Autodesk Inventor part; units mm, degrees
ref_plane "Work Plane1" through (0, 0, 26.65) normal (0, 0, 1) x (1, 0, 0)
ref_plane "YZ Plane" through (0, 0, 0) normal (1, 0, 0) x (0, 1, 0)
ref_plane "XZ Plane" through (0, 0, 0) normal (0, 1, 0) x (-1, 0, 0)
sketch "Sketch1" plane through (0, 0, 0) normal (1, 0, 0) x (0, 1, 0)
  line L0 (0, 0) -> (0, -22.65)
  line L1 (0, 0) -> (0, 26.65)
  line L2 (4, -26.65) -> (51, -26.65)
  arc A0 (0, -22.65) -> (4, -26.65) centre (4, -22.65) ccw
  point P0 (0, -26.65)
  dimension "d0" = 26.65
  dimension "d1" = 26.65
  dimension "d2" = 51
  dimension "d3" = 4
ref_plane "Work Plane1" through (0, 0, 26.65) normal (0, 0, 1) x (1, 0, 0)
sketch "Sketch2" plane through (0, 0, 26.65) normal (0, 0, 1) x (1, 0, 0)
  line L0 (-25, 1.5) -> (25, 1.5)
  line L1 (25, 1.5) -> (25, -1.5)
  line L2 (25, -1.5) -> (-25, -1.5)
  line L3 (-25, -1.5) -> (-25, 1.5)
  line L4 (-25, 1.5) -> (25, -1.5) construction
  line L5 (25, 1.5) -> (-25, -1.5) construction
  point P0 (0, 0)
  dimension "d4" = 50
  dimension "d5" = 3
sweep "Sweep1" add profiles "Sketch2" path "Sketch1"
sketch "Sketch3" plane through (25, 4, -28.15) normal (0, 0, -1) x (-1, 0, 0)
  line L0 (0, 47) -> (50, 47) construction
  line L1 (50, 0) -> (50, 47) construction
  circle A0 centre (25, 26.5) radius 11
  point P0 (25, -4)
  dimension "d8" = 22
  dimension "d9" = 20.5
  dimension "d10" = 25
extrude "Extrusion1" cut sketch "Sketch3" against normal blind 10
sketch "Sketch4" plane through (25, 4, -28.15) normal (0, 0, -1) x (-1, 0, 0)
  circle A0 centre (25, 26.5) radius 11 construction
  line L0 (50, 0) -> (50, 47) construction
  line L1 (0, 0) -> (0, 47) construction
  line L2 (0, 47) -> (50, 47) construction
  line L3 (0, 0) -> (50, 0) construction
  circle A1 centre (40.5, 42) radius 2
  line L4 (25, 26.5) -> (14, 26.5) construction
  circle A2 centre (25, 26.5) radius 11 construction
  line L5 (25, 26.5) -> (25, 15.5) construction
  circle A3 centre (9.5, 42) radius 2
  circle A4 centre (40.5, 11) radius 2
  circle A5 centre (9.5, 11) radius 2
  line L6 (25, 26.5) -> (40.5, 42) construction
  circle A6 centre (35.253, 36.753) radius 2
  circle A7 centre (14.747, 36.753) radius 2
  circle A8 centre (35.253, 16.247) radius 2
  circle A9 centre (14.747, 16.247) radius 2
  point P0 (25, -4)
  point P1 (33.8388, 35.3388)
  point P2 (32.7782, 34.2782)
  dimension "d17" = 4
  dimension "d13" = 4
  dimension "d14" = 15.5
  dimension "d15" = 15.5
  dimension "d18" = 1.5
extrude "Extrusion2" cut sketch "Sketch4" against normal blind 10
sketch "Sketch5" plane through (25, 4, -28.15) normal (0, 0, -1) x (-1, 0, 0)
  line L0 (0, 47) -> (50, 47) construction
  line L1 (50, 0) -> (50, 47) construction
  line L2 (0, 0) -> (0, 47) construction
  line L3 (0, 43.5) -> (5, 47)
  line L4 (25, 47) -> (25, 37.5) construction
  circle A0 centre (25, 26.5) radius 11 construction
  line L5 (50, 43.5) -> (45, 47)
  line L6 (0, 43.5) -> (0, 47)
  line L7 (0, 47) -> (5, 47)
  line L8 (45, 47) -> (50, 47)
  line L9 (50, 47) -> (50, 43.5)
  line L10 (50, 0) -> (50, 47)
  point P0 (25, -4)
  point P1 (0, 23.5)
  dimension "d21" = 20
  dimension "d22" = 20
extrude "Extrusion3" cut sketch "Sketch5" against normal blind 10
sketch "Sketch6" plane through (-25, 1.5, 26.65) normal (0, 1, 0) x (1, 0, 0)
  line L0 (0, 0) -> (0, 49.3) construction
  line L1 (0, 0) -> (50, 0) construction
  line L2 (50, 0) -> (50, 49.3) construction
  line L3 (45, 0) -> (50, 4.65)
  line L4 (25, 0) -> (25, 26.65) construction
  line L5 (5, 0) -> (0, 4.65)
  line L6 (5, 0) -> (0, 0)
  line L7 (0, 4.65) -> (0, 0)
  line L8 (45, 0) -> (50, 0)
  line L9 (50, 4.65) -> (50, 0)
  point P0 (50, 24.65)
  dimension "d25" = 20
  dimension "d26" = 20
extrude "Extrusion4" cut sketch "Sketch6" against normal blind 10
sketch "Sketch7" plane through (-25, 1.5, -22.65) normal (0, 1, 0) x (1, 0, 0)
  line L0 (10, -40.3) -> (10, -6.3) construction
  line L1 (12, -38.3) -> (12, -8.3)
  line L2 (8, -8.3) -> (8, -38.3)
  arc A0 (8, -38.3) -> (12, -38.3) centre (10, -38.3) ccw
  arc A1 (12, -8.3) -> (8, -8.3) centre (10, -8.3) ccw
  line L3 (11.5, 2.5) -> (7.5, 2.5) construction
  line L4 (0, -44.65) -> (0, 0) construction
  line L5 (45, -49.3) -> (5, -49.3) construction
  line L6 (25, -49.3) -> (25, -22.65) construction
  line L7 (38, -38.3) -> (38, -8.3)
  line L8 (42, -8.3) -> (42, -38.3)
  arc A2 (38, -38.3) -> (42, -38.3) centre (40, -38.3) ccw
  arc A3 (42, -8.3) -> (38, -8.3) centre (40, -8.3) ccw
  point P0 (10, -23.3)
  dimension "d29" = 34
  dimension "d30" = 4
  dimension "d31" = 8
  dimension "d32" = 9
extrude "Extrusion5" cut sketch "Sketch7" against normal blind 10
fillet "Fillet1" radius 1 8 edges at (20, 51, -26.65) (-20, 51, -26.65) (-25, 47.5, -26.65) (25, 47.5, -26.65) (25, 0, 22) (20, 0, 26.65) (-20, 0, 26.65) (-25, 0, 22)
sketch "Sketch8" plane through (-25, 4, -25.15) normal (-1, 0, 0) x (0, 0, 1)
  line L0 (0, 0) -> (0, 42.9793)
  arc A0 (0, 0) -> (2.5, -2.5) centre (2.5, 0) ccw
  line L1 (46.7144, -2.5) -> (2.5, -2.5)
  line L2 (10.8, -2.5) -> (40.8, -2.5)
  line L3 (0, 19.9793) -> (16.7144, -2.5)
  point P0 (25.15, -4)
  dimension "d36" = 30
  dimension "d37" = 23
extrude "Extrusion6" add sketch "Sketch8" against normal blind 2.5
mirror "Mirror1" about plane through (0, 0, 0) normal (1, 0, 0) of "Extrusion6"
properties part number "Stepper Bracket"
Can you work these out from the model? Positions are in its coordinate system, mm. A direction names the side the tool comes from. Give positions to 0.01 mm unless a question says otherwise; leave off trailing zeros. Order: outer loops, then holes, each group sorted by start corner. A loop starts at its lowest first (then second) coordinate and runs counter-clockwise, first axis right, second up. Notation, with made-up numbers: (-19.5, -10) - (14.5, -10) arc R33 cw to (14.5, 20) - close; hole circle Ø9 at (46.5, 10.5). An arc over 180 degrees is marked (long way). Use a Markdown table: item, result. Add a question column.
Q1. If we section it at D-D on y = 33: Write out the boundary of the cut face in (x, z).
Q2. If we section it at A-A on y = 46: Write out the boundary of the cut face in (x, z), plus the area to 3 significant figures.
Q3. Please list where these lines run through material, in increasing order: line 1 along X through (y, z) = (1, 0.5); line 2 along Y through (x, z) = (-15, -26); line 3 along Z through (x, y) = (-19.5, 30.5).
Q4. If we section it at B-B on z = 9.5: Write out the boundary of the cut face in (x, y).
Q5. If we mould it in two halves opening along X, with no side actions, what happens to faces 4 (the flat face through (-22.446, 49.288, -26.671)), 5 (the flat face through (-13, 0, 1)), 6 (the flat face through (0, 17, -28.15))? For each: released by +X, released by -X, zero draft, split by the parting line, or undercut.
Q6. If we section it at C-C on x = 18.5: Write out the boundary of the cut face in (y, z), plus the area to 3 significant figures.
Q7. I'm going to push flat-ended pins straight in: pin 1 (10 mm diameter, centred on x = -6.5, z = 16, fed in from +Y); pin 2 (3.5 mm diameter, centred on x = 15.5, y = 46, fed in from -Z); pin 3 (4.5 mm diameter, centred on x = 15.5, y = 15, fed in from +Z). Where does each tip first touch, or does it pass through?
Q8. On a 3-axis mill with a long thin cutter (end or side, diameter ignored), from which of +Z, -Z, +X, -X, +Y, -Y can I reach the whole of each face in a straight line? I mean faces 1 (the cylindrical face through (-0.315, 2.252, -24.437)), 2 (the cylindrical face through (14.96, 0.02, 17.65)), 3 (the flat face through (22.45, 0.02, 24.37)). Say none if no direction works.
Answers follow:
| question | item | result |
|---|---|---|
| 1 | outline | (-25, -28.15) - (-10.71, -28.15) - (-10.71, -25.15) - (-25, -25.15) - close; (10.71, -28.15) - (25, -28.15) - (25, -25.15) - (10.71, -25.15) - close |
| 2 | outline | (-25, -28.15) - (-17.5, -28.15) - (-17.5, -25.15) - (-25, -25.15) - close; (-13.5, -28.15) - (13.5, -28.15) - (13.5, -25.15) - (-13.5, -25.15) - close; (17.5, -28.15) - (25, -28.15) - (25, -25.15) - (17.5, -25.15) - close |
| 2 | area | 126 mm^2 |
| 3 | line 1 | x = -25 to -17, -13 to 13, 17 to 25 |
| 3 | line 2 | y = -0.36 to 13.06, 16.94 to 44.06, 47.94 to 51 |
| 3 | line 3 | z = -28.15 to -25.15 |
| 4 | outline | (-25, -1.5) - (-17, -1.5) - (-17, 1.5) - (-25, 1.5) - close; (-13, -1.5) - (13, -1.5) - (13, 1.5) - (-13, 1.5) - close; (17, -1.5) - (25, -1.5) - (25, 1.5) - (17, 1.5) - close |
| 5 | face 4 | released by -X |
| 5 | face 5 | undercut |
| 5 | face 6 | zero draft |
| 6 | outline | (-1.5, -22.65) arc R5.5 ccw to (4, -28.15) - (51, -28.15) - (51, -25.15) - (4, -25.15) arc R2.5 cw to (1.5, -22.65) - (1.5, 26.65) - (-1.5, 26.65) - close |
| 6 | area | 308 mm^2 |
| 7 | pin 1 | stops at y = 1.5 |
| 7 | pin 2 | passes through |
| 7 | pin 3 | stops at z = -25.15 |
| 8 | face 1 | +Z, +Y |
| 8 | face 2 | +Y, -Y |
| 8 | face 3 | +Z, +X, +Y, -Y |
